Verification items for the finished model (mm, model axes). Coordinates: 2 decimals unless noted, no trailing zeros. Write each loop counter-clockwise with the first axis right and the second up, starting at its lowest first coordinate (ties: lowest second). Pieces come first, ordered by that corner, then holes. Notation, with made-up numbers: (7, -10.75) -> (52, -10.75) arc R9 cw to (52, -6.75) -> close; hole circle Ø2 at (68.25, 15.25). An arc over 180 degrees is marked (long way). Use a Markdown table: item, result. Add a question column.
from build123d import *

# Parameters (mm, degrees)
SKETCH2_W           = 101.6
SKETCH2_H           = 101.6
SLEEVE_DEPTH        = 3.81
SKETCH3_R           = 2.54
HOLE_DEPTH          = 72.943005914
SKETCH4_R           = 46.99
SKETCH4_R_2         = 44.45
VINYL_OUTLINE_DEPTH = 1.27


with BuildPart() as part:
    # Sketch2 → Sleeve (new body)
    with BuildSketch(Plane.XY):
        Rectangle(SKETCH2_W, SKETCH2_H)
    extrude(amount=SLEEVE_DEPTH)

    # Sketch3 → Hole (cut, through all)
    with BuildSketch(Plane.XY.offset(3.81)):
        Circle(SKETCH3_R)
    extrude(amount=-HOLE_DEPTH, mode=Mode.SUBTRACT)

    # Sketch4 → Vinyl Outline (cut)
    with BuildSketch(Plane.XY.offset(3.81)):
        Circle(SKETCH4_R)
        Circle(SKETCH4_R_2, mode=Mode.SUBTRACT)
    extrude(amount=-VINYL_OUTLINE_DEPTH, mode=Mode.SUBTRACT)


solid = part.part
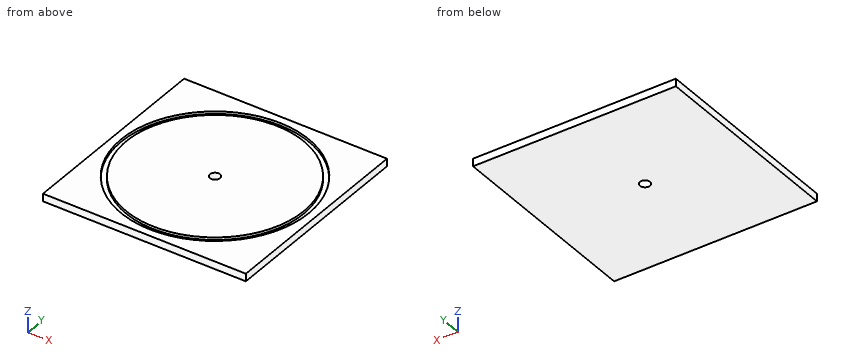
1) Cross-section at A-A on x = 0. Record the boundary of the cut face in (y, z).
2) Thickness scan on L1, parallel to Y at x = 0, z = 3.55; L2, parallel to Y at x = 0, z = 0.9; L3, parallel to Y at x = 12, z = 2.9. Record the ranges inside material, lowest first.
3) Cross-section at C-C on y = -42.5. Record the boundary of the cut face in (x, z).
4) Gauge pin test, flat ends, axial feed: pin 1 (3 mm diameter, centred on x = 0, y = 0, fed in from +Z); pin 2 (8 mm diameter, centred on x = -5, y = 11.5, fed in from -Z). Record the tip position at first contact, or that the pin passes through.
5) Cross-section at D-D on x = 18.5. Record the boundary of the cut face in (y, z), then the cut area to 3 significant figures.
Returned:
| question | item | result |
|---|---|---|
| 1 | outline | (-50.8, 0) -> (-2.54, 0) -> (-2.54, 3.81) -> (-44.45, 3.81) -> (-44.45, 2.54) -> (-46.99, 2.54) -> (-46.99, 3.81) -> (-50.8, 3.81) -> close; (2.54, 0) -> (50.8, 0) -> (50.8, 3.81) -> (46.99, 3.81) -> (46.99, 2.54) -> (44.45, 2.54) -> (44.45, 3.81) -> (2.54, 3.81) -> close |
| 2 | L1 | y = -50.8 to -46.99, -44.45 to -2.54, 2.54 to 44.45, 46.99 to 50.8 |
| 2 | L2 | y = -50.8 to -2.54, 2.54 to 50.8 |
| 2 | L3 | y = -50.8 to -45.43, -42.8 to 42.8, 45.43 to 50.8 |
| 3 | outline | (-50.8, 0) -> (50.8, 0) -> (50.8, 3.81) -> (20.05, 3.81) -> (20.05, 2.54) -> (13.02, 2.54) -> (13.02, 3.81) -> (-13.02, 3.81) -> (-13.02, 2.54) -> (-20.05, 2.54) -> (-20.05, 3.81) -> (-50.8, 3.81) -> close |
| 4 | pin 1 | passes through |
| 4 | pin 2 | stops at z = 0 |
| 5 | outline | (-50.8, 0) -> (50.8, 0) -> (50.8, 3.81) -> (43.2, 3.81) -> (43.2, 2.54) -> (40.42, 2.54) -> (40.42, 3.81) -> (-40.42, 3.81) -> (-40.42, 2.54) -> (-43.2, 2.54) -> (-43.2, 3.81) -> (-50.8, 3.81) -> close |
| 5 | area | 380 mm² |
